Model file for the job. Use its own axes, mm. A direction names the side the tool comes from. Round coordinates to 2 decimals unless told otherwise and drop trailing zeros. Order: outer loops, then holes, each group sorted by start corner. A loop starts at its lowest first (then second) coordinate and runs counter-clockwise, first axis right, second up. Notation, with made-up numbers: (60.5, 3.5) - (103.5, 3.5) arc R24 cw to (103.5, 21.5) - close; hole circle Ø4 at (10, 2). An arc over 180 degrees is marked (long way). Use one line per item in the form item = value.
from build123d import *

# Parameters (mm, degrees)
SKETCH_1_W          = 295
SKETCH_1_H          = 245
EXTRUDE_1_DEPTH     = 120
FILLET_1_R          = 10
SHELL_1_T           = -1.5
CUT_EXTRUDE_1_DEPTH = 342.220236797
SKETCH_3_W          = 150
SKETCH_3_H          = 60
CUT_EXTRUDE_2_DEPTH = 342.220236797
FILLET_2_R          = 10
FILLET_3_R          = 20
SKETCH_4_R          = 2.8
CUT_EXTRUDE_3_DEPTH = 10


with BuildPart() as part:
    # 草图1 → 凸台-拉伸1 (new body)
    with BuildSketch(Plane.XY):
        Rectangle(SKETCH_1_W, SKETCH_1_H)
    extrude(amount=EXTRUDE_1_DEPTH)

    # 圆角1
    fillet_1_edges = [part.edges().sort_by_distance(p)[0] for p in [
        (-147.5, 0, 120),
        (0, -122.5, 120),
        (147.5, 0, 120),
        (147.5, -122.5, 60),
        (-147.5, -122.5, 60),
        (-147.5, 122.5, 60),
        (147.5, 122.5, 60),
        (0, 122.5, 120),
    ]]
    fillet(fillet_1_edges, radius=FILLET_1_R)

    # 抽壳1
    shell_1_openings = [part.faces().sort_by_distance(p)[0] for p in [
        (0, 0, 0),
    ]]
    offset(amount=SHELL_1_T, openings=shell_1_openings, kind=Kind.INTERSECTION)

    # 草图2 → 切除-拉伸1 (cut, through all)
    with BuildSketch(Plane.ZY.offset(147.5)):
        with BuildLine():
            ThreePointArc((105, 0), (87.426406871, 42.426406871), (45, 60))
            Line((45, 60), (45, -60))
            ThreePointArc((45, -60), (87.426406871, -42.426406871), (105, 0))
        make_face()
        with BuildLine():
            Line((45, -60), (45, 60))
            ThreePointArc((45, 60), (20.313730334, 54.686269666), (0, 39.686269666))
            Line((0, 39.686269666), (0, -39.686269666))
            ThreePointArc((0, -39.686269666), (20.313730334, -54.686269666), (45, -60))
        make_face()
        with BuildLine():
            Line((0, -39.686269666), (0, 39.686269666))
            ThreePointArc((0, 39.686269666), (-15, 0), (0, -39.686269666))
        make_face()
        with BuildLine():
            Line((45, 60), (0, 60))
            Line((0, 60), (0, 39.686269666))
            ThreePointArc((0, 39.686269666), (20.313730334, 54.686269666), (45, 60))
        make_face()
        with BuildLine():
            Line((0, -39.686269666), (0, -60))
            Line((0, -60), (45, -60))
            ThreePointArc((45, -60), (20.313730334, -54.686269666), (0, -39.686269666))
        make_face()
    extrude(amount=-CUT_EXTRUDE_1_DEPTH, mode=Mode.SUBTRACT)

    # 草图3 → 切除-拉伸2 (cut, through all)
    with BuildSketch(Plane.ZY.offset(147.5)):
        with Locations((0, -60)):
            Rectangle(SKETCH_3_W, SKETCH_3_H)
        with Locations((0, 60)):
            Rectangle(SKETCH_3_W, SKETCH_3_H)
    extrude(amount=-CUT_EXTRUDE_2_DEPTH, mode=Mode.SUBTRACT)

    # 圆角2
    fillet_2_edges = [part.edges().sort_by_distance(p)[0] for p in [
        (146.75, 51.961524227, 75),
        (146.75, -51.961524227, 75),
        (146.75, -90, 0),
        (-146.75, -90, 0),
        (-146.75, -51.961524227, 75),
        (146.75, 90, 0),
        (-146.75, 90, 0),
        (-146.75, 51.961524227, 75),
    ]]
    fillet(fillet_2_edges, radius=FILLET_2_R)

    # 圆角3
    fillet_3_edges = [part.edges().sort_by_distance(p)[0] for p in [
        (146.75, -90, 75),
        (-146.75, -90, 75),
        (-146.75, 90, 75),
        (146.75, 90, 75),
    ]]
    fillet(fillet_3_edges, radius=FILLET_3_R)

    # 草图4 → 切除-拉伸3 (cut)
    with BuildSketch(Plane.XY.offset(120)):
        with Locations((-65, 0)):
            Circle(SKETCH_4_R)
        with Locations((65, 0)):
            Circle(SKETCH_4_R)
    extrude(amount=-CUT_EXTRUDE_3_DEPTH, mode=Mode.SUBTRACT)


solid = part.part
(1) Pin check, flat tips, straight feed: pin 1 (0.8 mm diameter, centred on x = 146.5, y = -66, fed in from -Z); pin 2 (3.5 mm diameter, centred on x = -65, y = 0, fed in from +Z); pin 3 (4 mm diameter, centred on x = -66, y = 42.5, fed in from -Z); pin 4 (6.5 mm diameter, centred on x = 65, y = 0, fed in from +Z). Stop position of each tip, or through.
Report:
pin_1 = 75
pin_2 = through
pin_3 = 118.5
pin_4 = 120
(2) Slice it at C-C on y = -43.5. Give the cut face in (x, z), then the cut area to 3 significant figures.
Report:
outline = (-147.5, 86.32) - (-146, 86.32) - (-146, 110) arc R8.5 cw to (-137.5, 118.5) - (137.5, 118.5) arc R8.5 cw to (146, 110) - (146, 86.32) - (147.5, 86.32) - (147.5, 110) arc R10 ccw to (137.5, 120) - (-137.5, 120) arc R10 ccw to (-147.5, 110) - close
area = 527 mm2
(3) Probe probe 1 along X at (y, z) = (-111.5, 76); probe 2 along Y at (x, z) = (-88, 58); probe 3 along Z at (x, y) = (3.5, -79). List the from-to ranges inside material, lowest first. Write a range as [from, to].
Report:
probe_1 = [-147.5, -146], [146, 147.5]
probe_2 = [-122.5, -121], [121, 122.5]
probe_3 = [118.5, 120]
(4) Pull direction X, two halves, no side cores. Call faces 1 (the face through (-146.74, -84.297, 68.986)), 2 (the face through (143.58, 118.44, 55.77)), 3 (the face through (144.65, 1.58, 116.99)): released by +X, released by -X, zero draft, split by the parting line, or undercut.
Report:
face_1 = zero draft
face_2 = undercut
face_3 = released by +X
(5) Slice it at D-D on z = 87. Give the cut face in (x, y), then the cut area to 3 significant figures.
Report:
outline = (-147.5, -112.5) arc R10 ccw to (-137.5, -122.5) - (137.5, -122.5) arc R10 ccw to (147.5, -112.5) - (147.5, -42.85) - (146, -42.85) - (146, -112.5) arc R8.5 cw to (137.5, -121) - (-137.5, -121) arc R8.5 cw to (-146, -112.5) - (-146, -42.85) - (-147.5, -42.85) - close; (-147.5, 42.85) - (-146, 42.85) - (-146, 112.5) arc R8.5 cw to (-137.5, 121) - (137.5, 121) arc R8.5 cw to (146, 112.5) - (146, 42.85) - (147.5, 42.85) - (147.5, 112.5) arc R10 ccw to (137.5, 122.5) - (-137.5, 122.5) arc R10 ccw to (-147.5, 112.5) - close
area = 1,330 mm2
(6) Slice it at A-A on z = 43. Give the cut face in (x, y).
Report:
outline = (-147.5, -112.5) arc R10 ccw to (-137.5, -122.5) - (137.5, -122.5) arc R10 ccw to (147.5, -112.5) - (147.5, -90) - (146, -90) - (146, -112.5) arc R8.5 cw to (137.5, -121) - (-137.5, -121) arc R8.5 cw to (-146, -112.5) - (-146, -90) - (-147.5, -90) - close; (-147.5, 90) - (-146, 90) - (-146, 112.5) arc R8.5 cw to (-137.5, 121) - (137.5, 121) arc R8.5 cw to (146, 112.5) - (146, 90) - (147.5, 90) - (147.5, 112.5) arc R10 ccw to (137.5, 122.5) - (-137.5, 122.5) arc R10 ccw to (-147.5, 112.5) - close
(7) Tool access for faces 4 (the face through (144.49, -119.65, 55.77)), 5 (the face through (-146.74, 92.85, 3.01)), 6 (the face through (1.93, -118.58, 115.94)): list every direction of +Z, -Z, +X, -X, +Y, -Y with a clear straight run to the whole face (end or side of a thin tool).
Report:
face_4 = +Z, -Z, +X, -Y
face_5 = -Z, +X, -X
face_6 = -Z
(8) Slice it at B-B on x = -103.5. Give the cut face in (y, z), then the cut area to 3 significant figures.
Report:
outline = (-122.5, 0) - (-121, 0) - (-121, 110) arc R8.5 cw to (-112.5, 118.5) - (112.5, 118.5) arc R8.5 cw to (121, 110) - (121, 0) - (122.5, 0) - (122.5, 110) arc R10 ccw to (112.5, 120) - (-112.5, 120) arc R10 ccw to (-122.5, 110) - close
area = 711 mm2
